Source: CAD feature listing. Evaluate the final solid. Frame: model axes, mm. Round coordinates to 2 decimals unless told otherwise and drop trailing zeros. Loops run counter-clockwise (first coordinate to the right, second up) from the corner with the lowest first, then second, coordinate; pieces in that order, holes last. Notation, with made-up numbers: (-20, 34.5) - (-7, 34.5) arc R33 cw to (-7, 66.5) - close; hole circle Ø8 at (54, 19.5). An arc over 180 degrees is marked (long way). One line per question, with ' | ' between items.
from build123d import *

# Parameters (mm, degrees)
EXTRUDE1_START = 2.54
SKETCH1_R      = 1.1
EXTRUDE1_DEPTH = 7.62
SKETCH3_R      = 0.25
FILLET1_R      = 1


with BuildPart() as part:
    # Sketch1 → Extrude1 (new body)
    with BuildSketch(Plane(origin=(0, 0, 0), x_dir=(0, 0, -1), z_dir=(1, 0, 0)).offset(EXTRUDE1_START)):
        with Locations((-1.1, 0)):
            Circle(SKETCH1_R)
    extrude(amount=EXTRUDE1_DEPTH)

    # Sweep1: sweep along a path in Sketch2
    with BuildLine(Plane(origin=(0, 0, 0), x_dir=(1, 0, 0), z_dir=(0, 1, 0))) as sweep1_path:
        Line((2.54, -1.1), (1, -1.1))
        ThreePointArc((1, -1.1), (0.292893219, -0.807106781), (0, -0.1))
        Line((0, -0.1), (0, 3))
    # Sketch3 → Sweep1 (sweep)
    with BuildSketch(Plane.ZY.offset(-2.54)):
        with Locations((1.1, 0)):
            Circle(SKETCH3_R)
    sweep(path=sweep1_path.line)

    # Fillet1
    # the kernel refuses this fillet: 1 mm, written as the material it takes off along each edge
    with BuildSketch(Plane(origin=(2.54, 0, 1.1), x_dir=(0, 0, -1), z_dir=(0, -1, 0))) as fillet1_piece_1:
        with BuildLine():
            CenterArc((0.1, 0.988685997), FILLET1_R, 278.626926559, 81.373073441)
            Line((0.25, 0), (0.253, -0.01977372))
            ThreePointArc((0.253, -0.01977372), (0.675, -0.02), (1.1, -0.02))
            Line((1.1, -0.02), (1.12, 0))
            Line((1.12, 0), (1.12, 0.988685997))
            Line((1.12, 0.988685997), (1.1, 0.988685997))
        make_face()
    revolve(axis=Axis((2.54, 0, 1.1), (1, 0, 0)), mode=Mode.SUBTRACT)

    # Mirror1: part across plane


with BuildPart() as part_1:
    add(part.part)
    add(part.part.mirror(Plane(origin=(10.16, 0, 1.1), x_dir=(0, 0, 1), z_dir=(1, 0, 0))))


solid = part_1.part
1. Section query C-C, the plane z = 0.3. Give the number of separate pieces and of enclosed holes in the cut face, plus the area to 3 significant figures.
Worked out:
separate pieces: 3 | enclosed holes: 0 | area: 22.1 mm2
2. Material intervals for probe 1 along X at (y, z) = (-0.1, 0.2); probe 2 along X at (y, z) = (0, -0.5); probe 3 along Z at (x, y) = (13.25, -0.45), sorted ascending.
Worked out:
probe 1: x = -0.23 to 0.24, 2.94 to 17.38, 20.08 to 20.55 | probe 2: x = -0.25 to 0.25, 20.07 to 20.57 | probe 3: z = 0.1 to 2.1
3. Section query A-A, the plane z = -0.65. Return loops of the section in (x, y).
Worked out:
outline: circle Ø0.5 at (0, 0); circle Ø0.5 at (20.32, 0)
4. Section query D-D, the plane x = 10. Return loops of the section in (y, z), plus the area to 3 significant figures.
Worked out:
outline: circle Ø2.2 at (0, 1.1) | area: 3.80 mm2
5. Section query B-B, the plane x = 19. Return loops of the section in (y, z), plus the area to 3 significant figures.
Worked out:
outline: circle Ø0.5 at (0, 1.1) | area: 0.196 mm2
